Input: part model. Units: mm. Frame: model coordinates. A direction names the side the tool comes from. Coordinates: 2 decimals unless noted, no trailing zeros. Write each loop counter-clockwise with the first axis right and the second up, starting at its lowest first coordinate (ties: lowest second). Pieces come first, ordered by that corner, then holes. Notation, with made-up numbers: (62.5, -9) -> (77.5, -9) arc R14 cw to (77.5, 6) -> close; hole circle Ø2 at (84.25, 34). An arc over 180 degrees is marked (long way). One line per question, with ' | ' between items. Start each with the question number.
```python
from build123d import *

# Parameters (mm, degrees)
EXTRUDE_1_DEPTH     = 60
SKETCH_2_W          = 5
SKETCH_2_H          = 8
EXTRUDE_2_DEPTH     = 197
CHAMFER_1_SIZE      = 20
CHAMFER_2_SIZE      = 2
SKETCH_4_W          = 85
SKETCH_4_H          = 8
CUT_EXTRUDE_1_DEPTH = 10
SKETCH_5_W          = 8
SKETCH_5_H          = 10
EXTRUDE_3_DEPTH     = 2


with BuildPart() as part:
    # 草图1 → 凸台-拉伸1 (new body)
    with BuildSketch(Plane.XY):
        Polygon((5.6, 10.6), (3.2, 10.6), (3.2, 15.2), (0, 15.2), (0, 0), (3.2, 0), (3.2, 4.6), (5.6, 4.6), (5.6, -2.4), (-2.4, -2.4), (-2.4, 17.6), (5.6, 17.6), align=None)
    extrude(amount=EXTRUDE_1_DEPTH)

    # 草图2 → 凸台-拉伸2 (add)
    with BuildSketch(Plane.ZY.offset(2.4)):
        with Locations((2.5, 7.6)):
            Rectangle(SKETCH_2_W, SKETCH_2_H)
    extrude(amount=EXTRUDE_2_DEPTH)

    # 倒角1
    chamfer_1_edges = [part.edges().sort_by_distance(p)[0] for p in [
        (-2.4, 7.6, 5),
    ]]
    chamfer(chamfer_1_edges, length=CHAMFER_1_SIZE)

    # 倒角2
    chamfer_2_edges = [part.edges().sort_by_distance(p)[0] for p in [
        (-2.4, 3.6, 15),
        (-2.4, 11.6, 15),
    ]]
    chamfer(chamfer_2_edges, length=CHAMFER_2_SIZE)

    # 草图4 → 切除-拉伸1 (cut)
    with BuildSketch(Plane(origin=(0, 0, 0), x_dir=(-1, 0, 0), z_dir=(0, 0, -1))):
        with Locations((156.9, 7.6)):
            Rectangle(SKETCH_4_W, SKETCH_4_H)
    extrude(amount=-CUT_EXTRUDE_1_DEPTH, mode=Mode.SUBTRACT)

    # 草图5 → 凸台-拉伸3 (add)
    with BuildSketch(Plane.ZY.offset(114.4)):
        with Locations((4, 7.6)):
            Rectangle(SKETCH_5_W, SKETCH_5_H)
    extrude(amount=-EXTRUDE_3_DEPTH)


solid = part.part
```
1) Section B-B, the plane x = -16. Return loops of the section in (y, z).
2) Section A-A, the plane z = 40. Return loops of the section in (x, y).
3) Access query for faces 4 (the face through (4, 10.6, 30)), 5 (the face through (-50.1, 3.6, 4.6)), 6 (the face through (2, 0, 30)). Directions: +Z, -Z, +X, -X, +Y, -Y. A direction counts if a zero-diameter tool reaches every point of the face in a straight line with its end or side. Return the directions, or none.
4) Pull-direction query (Y, two-part tool) for faces 1 (the face through (3.2, 2, 30)), 2 (the face through (-114.4, 8, 4)), 3 (the face through (2, 17.6, 30)); classes: released by +Y, released by -Y, zero draft, split by the parting line, or undercut.
5) Section C-C, the plane z = 15. Return loops of the section in (x, y).
6) Section D-D, the plane x = -29. Return loops of the section in (y, z).
7) First-contact query: P1, Ø1, axis at x = -113, z = 2, coming from the -Y side; P2, Ø2.5, axis at y = 3, z = 15.5, coming from the -X side; P3, Ø10, axis at y = 5, z = 41.5, coming from the +X side; P4, Ø6.5, axis at x = -50.5, y = 9, coming from the +Z side. Flat tips, straight axial feed; report the tip coordinate or a pass-through.
8) Ray query, line 1 (X direction, y = 4, z = 6.5); line 2 (X direction, y = 1.25, z = 9.5); line 3 (X direction, y = 15.5, z = 14). Return the intervals inside material, ascending.
Answer block:
1) outline: (3.6, 0) -> (11.6, 0) -> (11.6, 11.4) -> (3.6, 11.4) -> close
2) outline: (-2.4, -2.4) -> (5.6, -2.4) -> (5.6, 4.6) -> (3.2, 4.6) -> (3.2, 0) -> (0, 0) -> (0, 15.2) -> (3.2, 15.2) -> (3.2, 10.6) -> (5.6, 10.6) -> (5.6, 17.6) -> (-2.4, 17.6) -> close
3) face 4: +Z, -Z, +X | face 5: +Z, -Z, -Y | face 6: +Z, -Z
4) face 1: undercut | face 2: zero draft | face 3: released by +Y
5) outline: (-12.4, 3.6) -> (-4.4, 3.6) -> (-2.4, 1.6) -> (-2.4, -2.4) -> (5.6, -2.4) -> (5.6, 4.6) -> (3.2, 4.6) -> (3.2, 0) -> (0, 0) -> (0, 15.2) -> (3.2, 15.2) -> (3.2, 10.6) -> (5.6, 10.6) -> (5.6, 17.6) -> (-2.4, 17.6) -> (-2.4, 13.6) -> (-4.4, 11.6) -> (-12.4, 11.6) -> close
6) outline: (3.6, 0) -> (11.6, 0) -> (11.6, 5) -> (3.6, 5) -> close
7) P1: stops at y = 2.6 | P2: stops at x = -13 | P3: stops at x = 5.6 | P4: stops at z = 5
8) line 1: x = -114.4 to -112.4, -20.9 to 0, 3.2 to 5.6 | line 2: x = -2.4 to 0, 3.2 to 5.6 | line 3: x = -2.4 to 5.6
